from build123d import *

# Parameters (mm, degrees)
SKETCH1_W           = 62.6
SKETCH1_H           = 72.6
BOSS_EXTRUDE1_DEPTH = 24.14
SKETCH2_W           = 50
SKETCH2_H           = 24
BOSS_EXTRUDE2_DEPTH = 19
SKETCH3_W           = 62.6
SKETCH3_H           = 72.6
BOSS_EXTRUDE3_DEPTH = 7.3
FILLET1_R           = 2
FILLET2_R           = 11
SKETCH4_R           = 6.75
BOSS_EXTRUDE4_DEPTH = 15


with BuildPart() as part:
    # Sketch1 → Boss-Extrude1 (new body)
    with BuildSketch(Plane(origin=(0, 0, 0), x_dir=(1, 0, 0), z_dir=(0, 1, 0))):
        Rectangle(SKETCH1_W, SKETCH1_H)
    extrude(amount=BOSS_EXTRUDE1_DEPTH)

    # Sketch2 → Boss-Extrude2 (add)
    with BuildSketch(Plane.XZ):
        with Locations((0, -17.2)):
            Rectangle(SKETCH2_W, SKETCH2_H)
    extrude(amount=BOSS_EXTRUDE2_DEPTH)

    # Sketch3 → Boss-Extrude3 (add)
    with BuildSketch(Plane(origin=(0, 24.14, 0), x_dir=(1, 0, 0), z_dir=(0, 1, 0))):
        Rectangle(SKETCH3_W, SKETCH3_H)
    extrude(amount=BOSS_EXTRUDE3_DEPTH)

    # Fillet1
    fillet1_edges = [part.edges().sort_by_distance(p)[0] for p in [
        (0, 31.44, 36.3),
        (31.3, 31.44, 0),
        (0, 31.44, -36.3),
        (-31.3, 31.44, 0),
        (0, 0, 36.3),
        (-31.3, 0, 0),
        (0, 0, -36.3),
        (31.3, 0, 0),
        (31.3, 15.72, 36.3),
        (-31.3, 15.72, 36.3),
        (-31.3, 15.72, -36.3),
        (31.3, 15.72, -36.3),
    ]]
    fillet(fillet1_edges, radius=FILLET1_R)

    # Fillet2
    fillet2_edges = [part.edges().sort_by_distance(p)[0] for p in [
        (-25, -9.5, -5.2),
        (-25, -9.5, -29.2),
        (25, -9.5, -29.2),
        (25, -9.5, -5.2),
    ]]
    fillet(fillet2_edges, radius=FILLET2_R)

    # Sketch4 → Boss-Extrude4 (add)
    with BuildSketch(Plane.XY.offset(36.3)):
        with Locations((-14.64999991, 15.7200005)):
            Circle(SKETCH4_R)
        with Locations((14.64999991, 15.7200005)):
            Circle(SKETCH4_R)
    extrude(amount=BOSS_EXTRUDE4_DEPTH)


solid = part.part
Geometry check sheet. Reference: the model listing, model coordinates, mm. A direction names the side the tool comes from. Round coordinates to 2 decimals unless told otherwise and drop trailing zeros. Loops run counter-clockwise (first coordinate to the right, second up) from the corner with the lowest first, then second, coordinate; pieces in that order, holes last.
Item 1: Cross-section at A-A on y = 5. Record the boundary of the cut face in (x, z).
Item 2: Cross-section at C-C on y = 15.72. Record the boundary of the cut face in (x, z).
Item 3: Gauge pin test, flat ends, axial feed: pin 1 (9.5 mm diameter, centred on x = 3, y = -12.5, fed in from +Z); pin 2 (2 mm diameter, centred on y = -14, z = -17, fed in from +X); pin 3 (2 mm diameter, centred on y = -14, z = -17.5, fed in from -X). Record the tip position at first contact, or that the pin passes through.
Item 4: Mould release check, pull along X, two halves, no side actions. Record for faces 1 (the cylindrical face through (21.863, -9.633, -25.892)), 2 (the flat face through (0, 16, 36.3)), 3 (the cylindrical face through (0.41, 0.6, 35.73)): pulls with the +X half, pulls with the -X half, needs draft (parallel to the pull), parting line crosses it, or undercut.
Item 5: Thickness scan on line 1 (Z direction, x = 3.5, y = -13); line 2 (Y direction, x = 6, z = 9.5); line 3 (Z direction, x = 22.5, y = 24.5). Record the ranges inside material, lowest first.
Item 6: Cross-section at D-D on x = 12. Record the boundary of the cut face in (y, z), then the cut area to 3 significant figures.
Item 7: Cross-section at B-B on z = 29.5. Record the boundary of the cut face in (x, y).
Item 8: Access from +Z, -Z, +X, -X, +Y, -Y to the whole of each face (thin tool, end or side, straight path). Record for faces 4 (the cylindrical face through (-21.863, -9.633, -25.892)), 5 (the cylindrical face through (9.293, 11.613, 43.695)), 6 (the flat face through (0, -9, -29.2)), 7 (the flat face through (-25, -9, -17)).
Answer sheet:
1. outline: (-31.3, -34.3) arc R2 ccw to (-29.3, -36.3) - (29.3, -36.3) arc R2 ccw to (31.3, -34.3) - (31.3, 34.3) arc R2 ccw to (29.3, 36.3) - (-29.3, 36.3) arc R2 ccw to (-31.3, 34.3) - close
2. outline: (-31.3, -34.3) arc R2 ccw to (-29.3, -36.3) - (29.3, -36.3) arc R2 ccw to (31.3, -34.3) - (31.3, 34.3) arc R2 ccw to (29.3, 36.3) - (21.4, 36.3) - (21.4, 51.3) - (7.9, 51.3) - (7.9, 36.3) - (-7.9, 36.3) - (-7.9, 51.3) - (-21.4, 51.3) - (-21.4, 36.3) - (-29.3, 36.3) arc R2 ccw to (-31.3, 34.3) - close
3. pin 1: stops at z = -5.2
3. pin 2: stops at x = 25
3. pin 3: stops at x = -25
4. face 1: pulls with the +X half
4. face 2: undercut
4. face 3: needs draft
5. line 1: z = -29.2 to -5.2
5. line 2: y = 0 to 31.44
5. line 3: z = -36.3 to 36.3
6. outline: (-19, -29.2) - (0, -29.2) - (0, -34.3) arc R2 ccw to (2, -36.3) - (29.44, -36.3) arc R2 ccw to (31.44, -34.3) - (31.44, 34.3) arc R2 ccw to (29.44, 36.3) - (21.93, 36.3) - (21.93, 51.3) - (9.51, 51.3) - (9.51, 36.3) - (2, 36.3) arc R2 ccw to (0, 34.3) - (0, -5.2) - (-19, -5.2) - close
6. area: 2,920 mm2
7. outline: (-31.3, 2) arc R2 ccw to (-29.3, 0) - (29.3, 0) arc R2 ccw to (31.3, 2) - (31.3, 29.44) arc R2 ccw to (29.3, 31.44) - (-29.3, 31.44) arc R2 ccw to (-31.3, 29.44) - close
8. face 4: -Z, -X, -Y
8. face 5: +Z
8. face 6: -Z, +X, -X, -Y
8. face 7: +Z, -Z, -X, -Y
